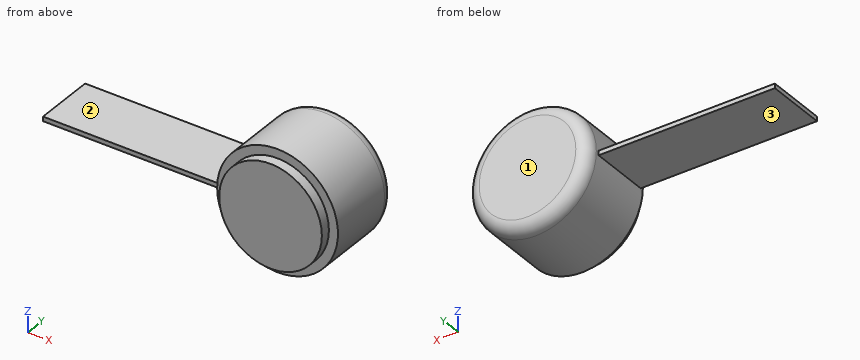
Autodesk Inventor part; units mm, degrees
ref_plane "XZ Plane" through (0, 0, 0) normal (0, 1, 0) x (-1, 0, 0)
ref_plane "XY Plane" through (0, 0, 0) normal (0, 0, 1) x (1, 0, 0)
sketch "Sketch2" plane through (0, 0, 0) normal (0, 1, 0) x (-1, 0, 0)
  circle A0 centre (0, 0) radius 20
  dimension "d0" = 40
extrude "Extrusion1" add sketch "Sketch2" along normal blind 26.1125
sketch "Sketch3" plane through (0, 0, 0) normal (0, -1, 0) x (1, 0, 0)
  circle A0 centre (0, 0) radius 20
  circle A1 centre (0, 0) radius 17
  dimension "d3" = 3
extrude "Extrusion2" add sketch "Sketch3" along normal blind 3.3375 contours A1
fillet "Fillet1" radius 4 1 edges at (20, 26.1125, 0)
ref_plane "Work Plane1" through (-20, 0, 0) normal (1, 0, 0) x (0, 1, 0)
sketch "Sketch4" plane through (-20, 0, 0) normal (1, 0, 0) x (0, 1, 0)
  line L0 (21, 0.75) -> (1, 0.75)
  line L1 (1, 0.75) -> (1, -0.75)
  line L2 (1, -0.75) -> (21, -0.75)
  line L3 (21, -0.75) -> (21, 0.75)
  point P0 (0, 0)
  dimension "d7" = 20
  dimension "d8" = 0.75
  dimension "d9" = 0.75
  dimension "d10" = 1
extrude "Extrusion3" add sketch "Sketch4" along normal blind 25.2375 and the other way blind 58.3375
properties part number "MagBallHolder"
CAD build for the part. Positions are in the model's coordinates, mm. Face numbers are marked on the shaded views. A direction names the side the tool comes from. Round coordinates to 2 decimals unless told otherwise and drop trailing zeros. Order: outer loops, then holes, each group sorted by start corner. A loop starts at its lowest first (then second) coordinate and runs counter-clockwise, first axis right, second up.
Item 1: Probe line 1 along X through (y, z) = (11.5, -10.5); line 2 along Z through (x, y) = (-22.5, 6.25); line 3 along X through (y, z) = (5, 12.5). List the from-to ranges inside material, lowest first.
Item 2: Tool access for the marked faces 1, 2 and 3: list every direction of +Z, -Z, +X, -X, +Y, -Y with a clear straight run to the whole face (end or side of a thin tool).
Item 3: Pin check, flat tips, straight feed: pin 1 (12 mm diameter, centred on x = -32.5, y = 6.5, fed in from +Z); pin 2 (0.8 mm diameter, centred on x = -61.5, z = 0, fed in from -Y); pin 3 (5 mm diameter, centred on x = -61, y = 20.5, fed in from -Z). Stop position of each tip, or through.
Item 4: Saw through at B-B on y = 3. Write the cut outline in (x, z), then the cut area to 3 significant figures.
Item 5: Saw through at A-A on x = 0. Write the cut outline in (y, z), then the cut area to 3 significant figures.
Reported:
1. line 1: x = -17.02 to 17.02
1. line 2: z = -0.75 to 0.75
1. line 3: x = -15.61 to 15.61
2. face 1: +Z, -Z, +X, -X, +Y
2. face 2: +Z, -X, +Y, -Y
2. face 3: -Z, -X, +Y, -Y
3. pin 1: stops at z = 0.75
3. pin 2: stops at y = 1
3. pin 3: stops at z = -0.75
4. outline: (-78.34, -0.75) - (-19.99, -0.75) arc R20 ccw (long way) to (-19.99, 0.75) - (-78.34, 0.75) - close
4. area: 1,340 mm2
5. outline: (-3.34, -17) - (0, -17) - (0, -20) - (22.11, -20) arc R4 ccw to (26.11, -16) - (26.11, 16) arc R4 ccw to (22.11, 20) - (0, 20) - (0, 17) - (-3.34, 17) - close
5. area: 1,150 mm2
